Model file for the job. Use its own axes, mm. Face numbers are marked on the shaded views. A direction names the side the tool comes from. Round coordinates to 2 decimals unless told otherwise and drop trailing zeros. Loops run counter-clockwise (first coordinate to the right, second up) from the corner with the lowest first, then second, coordinate; pieces in that order, holes last. Notation, with made-up numbers: M -37.75,50 L -4.75,50 A21 cw -4.75,80 Z; hole C 21.5,7.5 d6. An arc over 180 degrees is marked long. Answer in a Markdown table with one row per item.
from build123d import *

# Parameters (mm, degrees)
F0_R     = 12.858823
F0_W     = 19.820329
F0_H     = 20.111802
F1_DEPTH = 25.4
F2_W     = 25.504097
F2_H     = 17.488524
F3_DEPTH = 25.4


with BuildPart() as f1:
    # F0 (on Top) → F1 (new body)
    with BuildSketch(Plane.XY):
        Polygon((38.766231, 25.504097), (-39.057706, 25.504097), (-39.057706, -31.333605), (38.766231, -31.333605), (38.766231, 5.392295), align=None)
        with Locations((0, -2.914754)):
            Circle(F0_R, mode=Mode.SUBTRACT)
        with Locations((48.676395, 15.448196)):
            Rectangle(F0_W, F0_H)
    extrude(amount=F1_DEPTH)

    # F2 (on face) → F3 (join)
    with BuildSketch(Plane(origin=(-39.057706, 0, 0), x_dir=(0, -1, 0), z_dir=(-1, 0, 0))):
        with Locations((-12.752048, 40.369343)):
            Rectangle(F2_W, F2_H)
        Polygon((0, 31.625081), (-25.504097, 31.625081), (-25.504097, 0), (31.333605, 0), (31.333605, 31.625081), align=None)
    extrude(amount=F3_DEPTH)


solid = f1.part
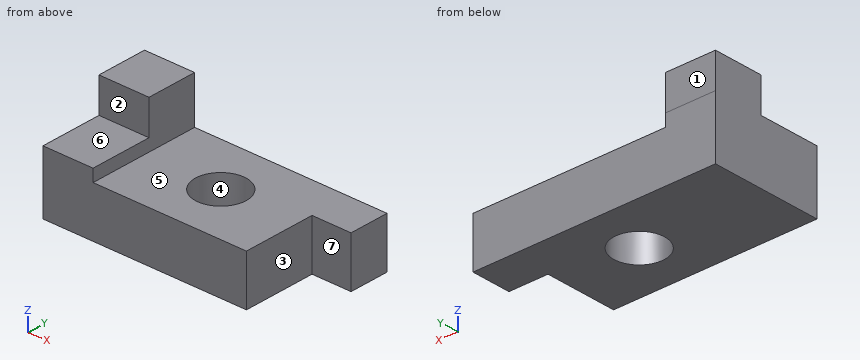
1. Saw through at A-A (x = 0). Write the cut outline in (y, z), and give its area (3 significant figures).
Verdict:
| item | result |
|---|---|
| outline | M -31.33,0 L -15.77,0 L -15.77,25.4 L -31.33,25.4 Z; M 9.94,0 L 25.5,0 L 25.5,25.4 L 9.94,25.4 Z |
| area | 790 mm² |
2. Wall check: probe 1 along Y at (x, z) = (0, 11.75); probe 2 along X at (y, z) = (-3, 16.5); probe 3 along Z at (x, y) = (-29.5, 6). Give the ranges that are in metal, low to high.
Verdict:
| item | result |
|---|---|
| probe 1 | y = -31.33 to -15.77, 9.94 to 25.5 |
| probe 2 | x = -64.46 to -12.86, 12.86 to 38.77 |
| probe 3 | z = 0 to 25.4 |
3. Saw through at D-D (y = -13). Write the cut outline in (x, z).
Verdict:
| item | result |
|---|---|
| outline | M -64.46,0 L -7.98,0 L -7.98,25.4 L -39.06,25.4 L -39.06,31.63 L -64.46,31.63 Z; M 7.98,0 L 38.77,0 L 38.77,25.4 L 7.98,25.4 Z |
4. Pin check, flat tips, straight feed: pin 1 (7.5 mm diameter, centred on x = -55.5, y = -9, fed in from +Z); pin 2 (12 mm diameter, centred on y = -15, z = 35.5, fed in from +X); pin 3 (7.5 mm diameter, centred on y = -8, z = 14, fed in from +X). Stop position of each tip, or through.
Verdict:
| item | result |
|---|---|
| pin 1 | stops at z = 31.63 |
| pin 2 | stops at x = -39.06 |
| pin 3 | stops at x = 38.77 |
5. Mould opens along Y. For the marked faces 1, 2, 3 and 4 say: +Y half, -Y half, draft (parallel to the pull), parting line (faces both ways), or undercut.
Verdict:
| item | result |
|---|---|
| face 1 | +Y half |
| face 2 | -Y half |
| face 3 | draft |
| face 4 | undercut |
6. Tool access for the marked faces 5, 6 and 7: list every direction of +Z, -Z, +X, -X, +Y, -Y with a clear straight run to the whole face (end or side of a thin tool).
Verdict:
| item | result |
|---|---|
| face 5 | +Z, +X, +Y, -Y |
| face 6 | +Z, +X, -X, -Y |
| face 7 | +Z, -Z, +X, -Y |
7. Saw through at B-B (y = 14). Write the cut outline in (x, z), and give its area (3 significant figures).
Verdict:
| item | result |
|---|---|
| outline | M -64.46,0 L 58.59,0 L 58.59,25.4 L -39.06,25.4 L -39.06,49.11 L -64.46,49.11 Z |
| area | 3,730 mm² |
8. Saw through at C-C (z = 18). Write the cut outline in (x, y), and give its area (3 significant figures).
Verdict:
| item | result |
|---|---|
| outline | M -64.46,-31.33 L 38.77,-31.33 L 38.77,5.39 L 58.59,5.39 L 58.59,25.5 L -64.46,25.5 Z; hole C 0,-2.91 d25.72 |
| area | 5,750 mm² |
